Check sheet for the modelled part. Datum: model origin and axes. Units: mm. A direction names the side the tool comes from. Round coordinates to 2 decimals unless told otherwise and drop trailing zeros. Loops run counter-clockwise (first coordinate to the right, second up) from the corner with the lowest first, then second, coordinate; pieces in that order, holes last. Notation, with made-up numbers: (16, 41) -> (70, 41) arc R30 cw to (70, 67) -> close; hole circle Ø2 at (-5.75, -11). An arc over 180 degrees is marked (long way). One line per question, with ' | ' between items.
```python
from build123d import *

# Parameters (mm, degrees)
F0_W      = 127
F0_H      = 127
F1_DEPTH  = 127
F4_DEPTH  = 88.9
F5_W      = 38.1
F5_H      = 88.9
F6_DEPTH  = 127
F7_W      = 38.1
F7_H      = 50.712608
F7_H_2    = 50.8
F8_DEPTH  = 93.98
F9_W      = 38.1
F9_H      = 93.98
F10_DEPTH = 12.7


with BuildPart() as f1:
    # F0 (on Top) → F1 (new body)
    with BuildSketch(Plane.XY):
        Rectangle(F0_W, F0_H)
    extrude(amount=F1_DEPTH)

    # F3 (on face) → F4 (cut)
    with BuildSketch(Plane.YZ.offset(63.5)):
        Polygon((-63.5, 127), (-63.5, 12.7), (25.4, 127), align=None)
    extrude(amount=-F4_DEPTH, mode=Mode.SUBTRACT)

    # F5 (on face) → F6 (join)
    with BuildSketch(Plane.XY.offset(127)):
        with Locations((44.45, -19.05)):
            Rectangle(F5_W, F5_H)
    extrude(amount=-F6_DEPTH)

    # F7 (on face) → F8 (cut)
    with BuildSketch(Plane.XY.offset(127)):
        with Locations((44.45, -38.143696)):
            Rectangle(F7_W, F7_H)
        with Locations((-44.45, -37.963312)):
            Rectangle(F7_W, F7_H_2)
    extrude(amount=-F8_DEPTH, mode=Mode.SUBTRACT)

    # F9 (on face) → F10 (cut)
    with BuildSketch(Plane.XZ.offset(63.5)):
        with Locations((-44.45, 80.01)):
            Rectangle(F9_W, F9_H)
    extrude(amount=-F10_DEPTH, mode=Mode.SUBTRACT)


solid = f1.part
```
(1) Set-up check for faces 4 (the face through (63.5, 13, 50)), 5 (the face through (-1, 1, 0)), 6 (the face through (-25.4, -23, 46)), 7 (the face through (44, -12.787, 81)), 8 (the face through (25.4, 2, 108)): record each of +Z, -Z, +X, -X, +Y, -Y from which the full face is reachable in a straight line by a thin tool's end or side.
Answer:
face 4: +Z, -Z, +X, +Y, -Y | face 5: -Z, +X, -X, +Y, -Y | face 6: +Z, -X, -Y | face 7: +Z, +X, -Y | face 8: +Z, -Y
(2) Scan lines: probe 1 along X at (y, z) = (-4, 100.5); probe 2 along Z at (x, y) = (-4.5, -24); probe 3 along Z at (x, y) = (-30.5, -56.5). Record each from-to range of solid material in increasing order.
Answer:
probe 1: x = -63.5 to -25.4, 25.4 to 63.5 | probe 2: z = 0 to 63.49 | probe 3: z = 0 to 33.02
(3) Mould release check, pull along X, two halves, no side actions. Record for faces 1 (the face through (-63.5, 13, 48)), 2 (the face through (0.36, -19.67, 69.05)), 3 (the face through (44, -38, 33.02)): +X half, -X half, draft (parallel to the pull), parting line (faces both ways), or undercut.
Answer:
face 1: -X half | face 2: undercut | face 3: draft
(4) Sectioned sample at A-A, the plane y = -35.5. Record the cut outline in (x, z).
Answer:
outline: (-63.5, 0) -> (63.5, 0) -> (63.5, 33.02) -> (25.4, 33.02) -> (25.4, 48.7) -> (-25.4, 48.7) -> (-25.4, 33.02) -> (-63.5, 33.02) -> close
(5) Go/stop test with flat-tipped pins: pin 1 (11.5 mm diameter, centred on x = -48.5, y = -32, fed in from +Z); pin 2 (6 mm diameter, centred on x = 32, y = 4, fed in from -Z); pin 3 (11.5 mm diameter, centred on x = -47.5, z = 70, fed in from -Y); pin 4 (10 mm diameter, centred on x = 15, z = 56.5, fed in from -Y). Record where each tip stops, or that it passes through.
Answer:
pin 1: stops at z = 33.02 | pin 2: stops at z = 0 | pin 3: stops at y = -12.56 | pin 4: stops at y = -33.32
(6) Sectioned sample at C-C, the plane z = 89. Record the cut outline in (x, y), and give its area (3 significant figures).
Answer:
outline: (-63.5, -12.56) -> (-25.4, -12.56) -> (-25.4, -4.16) -> (25.4, -4.16) -> (25.4, -12.79) -> (63.5, -12.79) -> (63.5, 63.5) -> (-63.5, 63.5) -> close | area: 9,240 mm2
(7) Sectioned sample at D-D, the plane x = 50. Record the cut outline in (y, z), and give its area (3 significant figures).
Answer:
outline: (-63.5, 0) -> (63.5, 0) -> (63.5, 127) -> (-12.79, 127) -> (-12.79, 33.02) -> (-63.5, 33.02) -> close | area: 11,400 mm2
(8) Sectioned sample at B-B, the plane x = 13. Record the cut outline in (y, z), and give its area (3 significant figures).
Answer:
outline: (-63.5, 0) -> (63.5, 0) -> (63.5, 127) -> (25.4, 127) -> (-63.5, 12.7) -> close | area: 11,000 mm2
